Can you work these out from the model? Positions are in its coordinate system, mm. A direction names the side the tool comes from. Round coordinates to 2 decimals unless told otherwise and drop trailing zeros. Order: outer loops, then holes, each group sorted by start corner. A loop starts at its lowest first (then second) coordinate and runs counter-clockwise, first axis right, second up.
from build123d import *

# Parameters (mm, degrees)
SKETCH1_R           = 3.5
SKETCH1_R_2         = 1.95
SKETCH1_R_3         = 1.475
SKETCH1_R_4         = 1.975
BOSS_EXTRUDE2_DEPTH = 5


with BuildPart() as part:
    # Sketch1 → Boss-Extrude2 (new body)
    with BuildSketch(Plane(origin=(0, 0, 0), x_dir=(1, 0, 0), z_dir=(0, 1, 0))):
        with BuildLine():
            Line((76.836482479, 56.919157308), (76.836482479, -60.080842545))
            ThreePointArc((76.836482479, -60.080842545), (74.932676609, -64.677036718), (70.336482479, -66.580842692))
            Line((70.336482479, -66.580842692), (-68.163517521, -66.580842545))
            ThreePointArc((-68.163517521, -66.580842545), (-133.166606879, -1.580842619), (-68.163517521, 63.419157308))
            Line((-68.163517521, 63.419157308), (70.336482479, 63.419157308))
            ThreePointArc((70.336482479, 63.419157308), (74.932676557, 61.515351386), (76.836482479, 56.919157308))
        make_face()
        with Locations(Location((18.836482479, 40.919291459, 0), (0, 0, 270))):
            Circle(SKETCH1_R, mode=Mode.SUBTRACT)
        with Locations(Location((51.836482479, 38.419157308, 0), (0, 0, 270))):
            Circle(SKETCH1_R_2, mode=Mode.SUBTRACT)
        with Locations(Location((68.836482479, 40.919291459, 0), (0, 0, 270))):
            Circle(SKETCH1_R, mode=Mode.SUBTRACT)
        with Locations(Location((70.336482479, 56.919157308, 0), (0, 0, 270))):
            Circle(SKETCH1_R_3, mode=Mode.SUBTRACT)
        with Locations(Location((18.836482479, -40.800748124, 0), (0, 0, 90))):
            Circle(SKETCH1_R, mode=Mode.SUBTRACT)
        with Locations(Location((70.336482479, -60.080842692, 0), (0, 0, 90))):
            Circle(SKETCH1_R_3, mode=Mode.SUBTRACT)
        with Locations(Location((51.685487167, -41.580700194, 0), (0, 0, 90))):
            Circle(SKETCH1_R_2, mode=Mode.SUBTRACT)
        with Locations(Location((68.836482479, -44.080708541, 0), (0, 0, 90))):
            Circle(SKETCH1_R, mode=Mode.SUBTRACT)
        with Locations(Location((-68.163517521, 56.919157308, 0), (0, 0, 270))):
            Circle(SKETCH1_R_3, mode=Mode.SUBTRACT)
        with Locations(Location((-98.163517521, 38.419157308, 0), (0, 0, 270))):
            Circle(SKETCH1_R_2, mode=Mode.SUBTRACT)
        with Locations(Location((-68.163517521, 18.109648094, 0), (0, 0, 270))):
            Circle(SKETCH1_R_4, mode=Mode.SUBTRACT)
        with Locations(Location((-68.163517521, -17.890351906, 0), (0, 0, 90))):
            Circle(SKETCH1_R_4, mode=Mode.SUBTRACT)
        with Locations(Location((-98.163517521, -40.000000036, 0), (0, 0, 90))):
            Circle(SKETCH1_R_2, mode=Mode.SUBTRACT)
        with Locations(Location((-68.163517521, -60.080842545, 0), (0, 0, 90))):
            Circle(SKETCH1_R_3, mode=Mode.SUBTRACT)
        with Locations(Location((-126.663517521, -1.580842619, 0), (0, 0, 270))):
            Circle(SKETCH1_R_3, mode=Mode.SUBTRACT)
        with BuildLine():
            Line((-31.663517521, 3.419157346), (19.336482479, 3.419157346))
            ThreePointArc((19.336482479, 3.419157346), (24.121172968, -1.796152166), (18.905863456, -6.580842654))
            Line((18.905863456, -6.580842654), (-32.094136544, -6.580842654))
            ThreePointArc((-32.094136544, -6.580842654), (-36.878827032, -1.365533142), (-31.663517521, 3.419157346))
        make_face(mode=Mode.SUBTRACT)
        with BuildLine():
            Line((-23.163517274, 21.419157346), (1.836482479, 21.419157346))
            ThreePointArc((1.836482479, 21.419157346), (6.836482479, 16.419157346), (1.836482479, 11.419157346))
            Line((1.836482479, 11.419157346), (-23.163517274, 11.419157346))
            ThreePointArc((-23.163517274, 11.419157346), (-28.163517274, 16.419157346), (-23.163517274, 21.419157346))
        make_face(mode=Mode.SUBTRACT)
        with BuildLine():
            Line((-23.166606879, -25.419653269), (1.833393121, -25.419653269))
            ThreePointArc((1.833393121, -25.419653269), (6.833393121, -20.419653269), (1.833393121, -15.419653269))
            Line((1.833393121, -15.419653269), (-23.166606879, -15.419653269))
            ThreePointArc((-23.166606879, -15.419653269), (-26.786365539, -20.419653269), (-23.166606879, -25.419653269))
        make_face(mode=Mode.SUBTRACT)
    extrude(amount=BOSS_EXTRUDE2_DEPTH)


solid = part.part
(1) I want a section at A-A, the plane y = 1.95. Give the number of separate pieces and of enclosed holes in the cut face, plus the area to 3 significant figures.
(2) I want a section at B-B, the plane z = -50. List the corners of the cut face in (x, y) for me.
(3) I want a section at C-C, the plane x = -117. List the corners of the cut face in (y, z) for me.
(4) On a 3-axis mill with a long thin cutter (end or side, diameter ignored), from which of +Z, -Z, +X, -X, +Y, -Y can I reach the whole of each face in a straight line? I mean faces 1 (the face through (-27, 0, 15)), 2 (the face through (-11, 2, -21.419)). Say none if no direction works.
(5) If we mould it in two halves opening along X, with no side actions, what happens to faces 3 (the face through (-133.15, 2.46, 3.01)), 4 (the face through (-28.162, 2.465, -16.309)), 5 (the face through (2, 2, 66.581)), 6 (the face through (-66.498, 2.465, -17.048))? For each: pulls with the +X half, pulls with the -X half, needs draft (parallel to the pull), parting line crosses it, or undercut.
(6) Please list where these lines run through material, in increasing order: probe 1 along Z at (x, y) = (-13, 3); probe 2 along Z at (x, y) = (68, 0.5); probe 3 along X at (y, z) = (4, 2).
Ans:
1. separate pieces: 1
1. enclosed holes: 18
1. area: 24,000 mm2
2. outline: (-107.72, 0) - (76.84, 0) - (76.84, 5) - (-107.72, 5) - close
3. outline: (0, -41.32) - (5, -41.32) - (5, 44.48) - (0, 44.48) - close
4. face 1: +Z, -Z, +X, -X, -Y
4. face 2: +Y, -Y
5. face 3: pulls with the -X half
5. face 4: undercut
5. face 5: needs draft
5. face 6: undercut
6. probe 1: z = -63.42 to -21.42, -11.42 to -3.42, 6.58 to 15.42, 25.42 to 66.58
6. probe 2: z = -63.42 to -44.32, -37.52 to 40.68, 47.48 to 66.58
6. probe 3: x = -133.17 to -128.08, -125.25 to -36.87, 24.11 to 76.84
